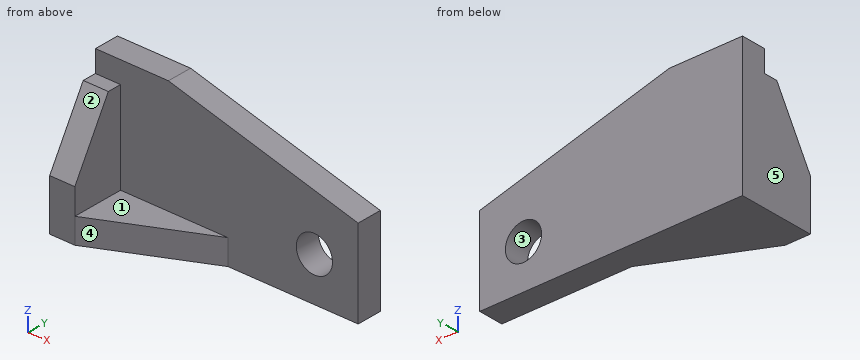
```python
from build123d import *

# Parameters (mm, degrees)
F0_R        = 7.874
F1_DEPTH    = 10.922
F2_DEPTH    = 33.528
F0_W        = 10.922
F0_H        = 19.3979742137
F3_DEPTH    = 33.528
F4_SIZE2    = 16.5711074263
F4_SIZE     = 28.702
F5_T4_DEPTH = 283.3190140635


# Not quite as in the source:
# - a fillet or chamfer that OpenCascade refuses, or shapes differently, is made with other operations: its cross-section is extruded or revolved along the edge and cut away or added


with BuildPart() as f1:
    # F0 (on Front) → F1 (new body)
    with BuildSketch(Plane.XZ):
        Polygon((-43.8717590123, 47.7630699762), (-75.6217590123, 47.7630699762), (-75.6217590123, 38.3650699762), (-64.6997590123, 38.3650699762), (-64.6997590123, 18.9670957625), (-64.6997590123, -1.5129300238), (-12.1217590123, -1.5129300238), (-12.1217590123, -12.4349300238), (38.6782409877, -12.4349300238), (38.6782409877, 25.643864141), align=None)
        with Locations((19.6282409877, 6.6150699762)):
            Circle(F0_R, mode=Mode.SUBTRACT)
    extrude(amount=F1_DEPTH)

    # F0 (on Front) → F2 (join)
    with BuildSketch(Plane.XZ):
        Polygon((-43.8717590123, -12.4349300238), (-12.1217590123, -12.4349300238), (-12.1217590123, -1.5129300238), (-64.6997590123, -1.5129300238), (-64.6997590123, -12.4349300238), align=None)
    extrude(amount=F2_DEPTH)

    # F0 (on Front) → F3 (join)
    with BuildSketch(Plane.XZ):
        with Locations((-70.1607590123, 28.6660828693)):
            Rectangle(F0_W, F0_H)
        Polygon((-64.6997590123, 18.9670957625), (-75.6217590123, 18.9670957625), (-75.6217590123, -12.4349300238), (-64.6997590123, -12.4349300238), (-64.6997590123, -1.5129300238), align=None)
    extrude(amount=F3_DEPTH)

    # F4
    f4_edges = [f1.edges().sort_by_distance(p)[0] for p in [
        (-70.160759, -33.528, 38.36507),
    ]]
    f4_side = f1.faces().sort_by_distance((-70.160759, -33.528, 37.551873))[0]
    chamfer(f4_edges, length=F4_SIZE, length2=F4_SIZE2, reference=f4_side)

    # F5: chamfer of 25.4 x 52.578 on 1 edges, made by hand


with BuildPart() as f5_tool2:
    # F5_s3 → F5_t4 (new body)
    with BuildSketch(Plane.XY.offset(-148.6334370556)):
        Polygon((-64.6997590123, -33.528), (-12.1217590123, -8.128), (-12.1217590123, -33.528), align=None)
    extrude(amount=F5_T4_DEPTH)

    split(bisect_by=Plane.XZ.offset(10.922), keep=Keep.TOP)


with BuildPart() as f1_1:
    add(f1.part)

    # F5_t1: cut F5_tool2
    add(f5_tool2.part, mode=Mode.SUBTRACT)


solid = f1_1.part
```
Could you check a few things on this model? Use its own coordinates, in mm. Face numbers are marked on the shaded views. A direction names the side the tool comes from. Round coordinates to 2 decimals unless told otherwise and drop trailing zeros. Loops run counter-clockwise (first coordinate to the right, second up) from the corner with the lowest first, then second, coordinate; pieces in that order, holes last. Notation, with made-up numbers: (-11, 42) - (42, 42) arc R20 cw to (42, 78) - close; hole circle Ø6 at (50.5, 20.25). An arc over 180 degrees is marked (long way). Answer as CSV lines item,"result".
1. I want a section at C-C on y = -27.5. List the corners of the cut face in (x, z) for me.
Filled in:
outline,"(-75.62, -12.43) - (-52.22, -12.43) - (-52.22, -1.51) - (-64.7, -1.51) - (-64.7, 20.1) - (-75.62, 20.1) - close"
2. For pin 1 Ø18 at (y, z) = (-20.5, 13.5) entering from +X; pin 2 Ø18 at (x, z) = (19.63, 6.62) entering from -Y; pin 3 Ø11.5 at (x, y) = (-51, -17) entering from +Z, each with a flat end and sliding along its axis, tell me the tip position at first contact or that it passes through.
Filled in:
pin 1,"stops at x = -64.7"
pin 2,"stops at y = -10.92"
pin 3,"stops at z = -1.51"
3. I want a section at B-B on z = -8. List the corners of the cut face in (x, y) for me.
Filled in:
outline,"(-75.62, -33.53) - (-64.7, -33.53) - (-17.91, -10.92) - (38.68, -10.92) - (38.68, 0) - (-75.62, 0) - close"
4. I want a section at A-A on x = 22.5. List the corners of the cut face in (y, z) for me, then the cut area to 3 significant figures.
Filled in:
outline,"(-10.92, -12.43) - (0, -12.43) - (0, -0.72) - (-10.92, -0.72) - close; (-10.92, 13.95) - (0, 13.95) - (0, 29.98) - (-10.92, 29.98) - close"
area,"303 mm^2"
5. On a 3-axis mill with a long thin cutter (end or side, diameter ignored), from which of +Z, -Z, +X, -X, +Y, -Y can I reach the whole of each face in a straight line? I mean the marked faces 1 and 2. Say none if no direction works.
Filled in:
face 1,"+Z, +X, -Y"
face 2,"+Z, +X, -X, -Y"
6. I want a section at D-D on y = -8.5. List the corners of the cut face in (x, z) for me.
Filled in:
outline,"(-75.62, -12.43) - (38.68, -12.43) - (38.68, 25.64) - (-43.87, 47.76) - (-75.62, 47.76) - close; hole circle Ø15.75 at (19.63, 6.62)"
7. Please list where these lines run through material, in increasing order: line 1 along Y through (x, z) = (3, 32); line 2 along X through (y, z) = (-22, 29); line 3 along Z through (x, y) = (-47, -23). Write a range as [from, to].
Filled in:
line 1,"y = [-10.92, 0]"
line 2,"x = [-75.62, -64.7]"
line 3,"z = [-12.43, -1.51]"
8. We'd pull the mould along X, two halves only. Please class the marked faces 3, 4 and 5: +X half, -X half, draft (parallel to the pull), parting line (faces both ways), or undercut.
Filled in:
face 3,"undercut"
face 4,"+X half"
face 5,"-X half"
